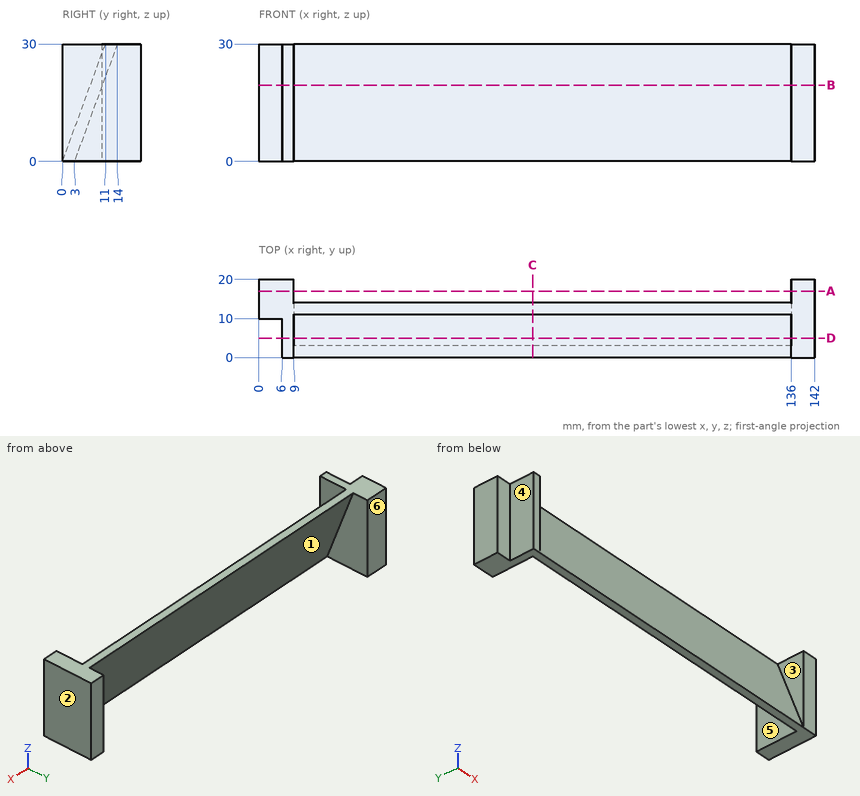
The drawing under review shows one solid part. Ordinate dimensions are in mm from its lowest x, y, z. A direction names the side the tool comes from. Coordinates: 2 decimals unless noted, no trailing zeros. Write each loop counter-clockwise with the first axis right and the second up, starting at its lowest first coordinate (ties: lowest second). Pieces come first, ordered by that corner, then holes. Notation, with made-up numbers: (18, -30.75) -> (63, -30.75) arc R24 cw to (63, 8.25) -> close; hole circle Ø2 at (13, -16.75). An arc over 180 degrees is marked (long way). One line per item, written item: value. Start each with the question number.
Q1. Add section D-D, the plane y = 5. Give the boundary of the cut face in (x, z), then the cut area to 3 significant figures.
Q2. For the marked faces 1, 2 and 3, list the 3-axis set-ups (+Z, -Z, +X, -X, +Y, -Y) from which the entire face can be reached by the end or side of a thin tool; tool diameter is ignored.
Q3. Clearance check with flat-ended pins moving along their axes: P1, Ø3, axis at x = 3.5, z = 17, coming from the -Y side; P2, Ø8, axis at y = 3.5, z = 15.5, coming from the -X side; P3, Ø5, axis at x = 107.5, z = 4, coming from the +Y side. State where each tip first meets the part, or that it passes through.
Q4. Add section C-C, the plane x = 70. Give the boundary of the cut face in (y, z), then the cut area to 3 significant figures.
Q5. Add section A-A, the plane y = 17. Give the boundary of the cut face in (x, z), then the cut area to 3 significant figures.
Q6. To check wall thickness, follow probe 1 along X at (y, z) = (4.25, 15.5); probe 2 along X at (y, z) = (12.25, 7); probe 3 along Y at (x, z) = (97.5, 26). State the ranges of each line that lie inside material, in increasing order.
Q7. The part is to be moulded in two halves that separate along X. For the marked faces 4, 5 and 6, say which applies: +X half, -X half, draft (parallel to the pull), parting line (faces both ways), or undercut.
Q8. Add section B-B, the plane z = 19.5. Give the boundary of the cut face in (x, y).
Response:
1. outline: (6, 0) -> (9, 0) -> (9, 5.45) -> (136, 5.45) -> (136, 0) -> (142, 0) -> (142, 30) -> (136, 30) -> (136, 13.64) -> (9, 13.64) -> (9, 30) -> (6, 30) -> close
1. area: 1,310 mm²
2. face 1: -Z, +Y
2. face 2: +Z, -Z, +X, +Y, -Y
2. face 3: +Z, -Y
3. P1: y = 10
3. P2: x = 6
3. P3: y = 5.38
4. outline: (0, 0) -> (3, 0) -> (14, 30) -> (11, 30) -> close
4. area: 90.0 mm²
5. outline: (0, 0) -> (9, 0) -> (9, 30) -> (0, 30) -> close; (136, 0) -> (142, 0) -> (142, 30) -> (136, 30) -> close
5. area: 450 mm²
6. probe 1: 6 to 9, 136 to 142
6. probe 2: 0 to 9, 136 to 142
6. probe 3: 9.53 to 12.53
7. face 4: -X half
7. face 5: undercut
7. face 6: draft
8. outline: (0, 10) -> (6, 10) -> (6, 0) -> (9, 0) -> (9, 7.15) -> (136, 7.15) -> (136, 0) -> (142, 0) -> (142, 20) -> (136, 20) -> (136, 10.15) -> (9, 10.15) -> (9, 20) -> (0, 20) -> close
